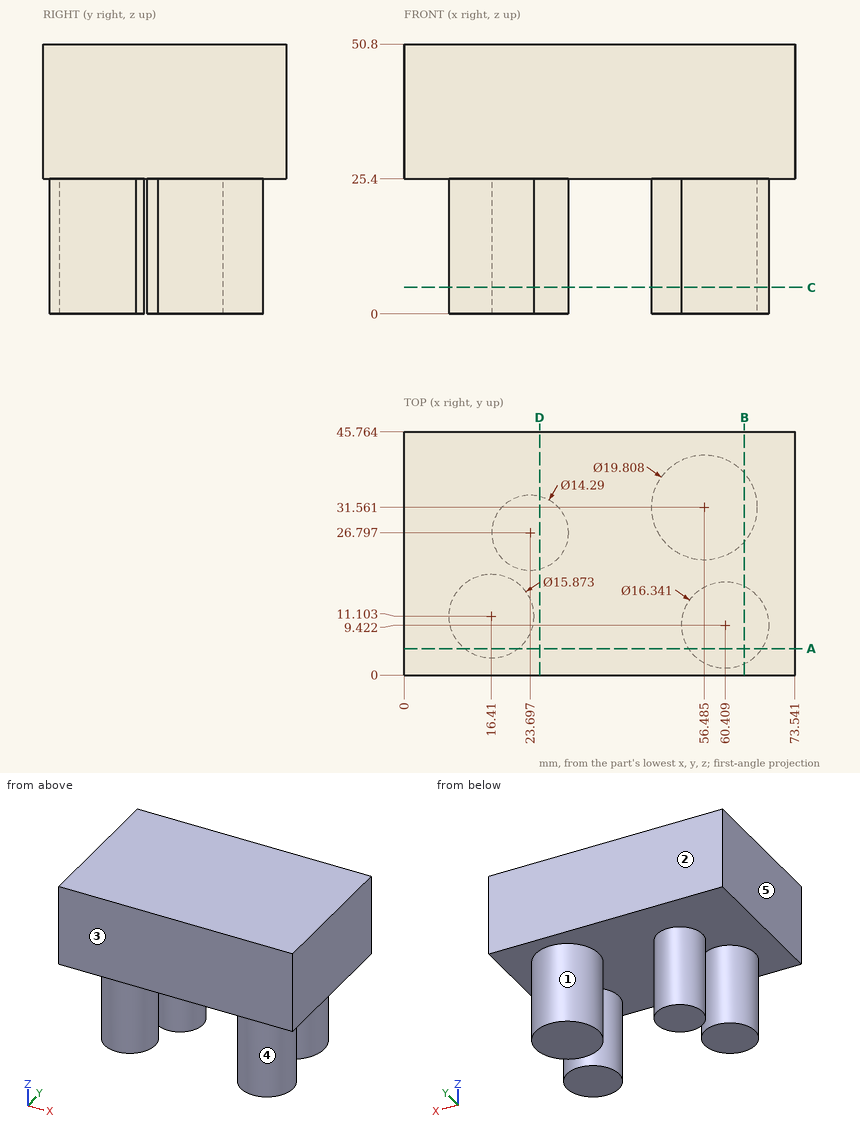
Geometry check sheet. Reference: drawing and pictorial views, mm from the part's lowest x, y, z. A direction names the side the tool comes from. Give positions to 0.01 mm unless a question says otherwise; leave off trailing zeros. Order: outer loops, then holes, each group sorted by start corner. A loop starts at its lowest first (then second) coordinate and runs counter-clockwise, first axis right, second up. Notation, with made-up numbers: M 45.5,-18.5 L 64.5,-18.5 A29 cw 64.5,7.5 Z; hole C 26.5,-10 d4. An arc over 180 degrees is marked long. Answer as a JSON object with one key per item and string values. Group by question number.
1) Scan lines: line 1 along Z through (x, y) = (12.5, 22.5); line 2 along X through (y, z) = (2, 20) (1 decimal); line 3 along X through (y, z) = (32.5, 13.5) (1 decimal). Record each from-to range of solid material in increasing order. Write a range as [from, to].
2) Access from +Z, -Z, +X, -X, +Y, -Y to the whole of each face (thin tool, end or side, straight path). Record for the marked faces 1 and 2.
3) Cross-section at B-B (x = 64). Enter the section's corners in (y, z) (1 decimal), then the cut area to 3 significant figures.
4) Cross-section at A-A (y = 5). Enter the section's corners in (x, z).
5) Depth check by flat-ended pin: pin 1 Ø6 at (y, z) = (11, 8.5) entering from +X; pin 2 Ø10 at (y, z) = (33.5, 10.5) entering from +X; pin 3 Ø12 at (x, z) = (58.5, 15.5) entering from -Y; pin 4 Ø3 at (y, z) = (36, 26.5) entering from -X. Enter the tip coordinate at first touch or a pass-through.
6) Cross-section at C-C (z = 5). Enter the section's corners in (x, y) (1 decimal), then the cut area to 3 significant figures.
7) Cross-section at D-D (x = 25.5). Enter the section's corners in (y, z) (1 decimal), then the cut area to 3 significant figures.
8) Mould release check, pull along X, two halves, no side actions. Record for the marked faces 3, 4 and 5: released by +X, released by -X, zero draft, split by the parting line, or undercut.
Result sheet:
{
 "1": {"line 1": "z = [25.4, 50.8]", "line 2": "x = [57, 63.8]", "line 3": "x = [19.4, 28], [46.6, 66.3]"},
 "2": {"face 1": "-Z", "face 2": "+Z, -Z, +X, -X, +Y"},
 "3": {"outline": "M 0,25.4 L 2.1,25.4 L 2.1,0 L 16.8,0 L 16.8,25.4 L 25.1,25.4 L 25.1,0 L 38,0 L 38,25.4 L 45.8,25.4 L 45.8,50.8 L 0,50.8 Z", "area": "1,860 mm2"},
 "4": {"outline": "M 0,25.4 L 11.34,25.4 L 11.34,0 L 21.48,0 L 21.48,25.4 L 53.54,25.4 L 53.54,0 L 67.28,0 L 67.28,25.4 L 73.54,25.4 L 73.54,50.8 L 0,50.8 Z"},
 "5": {"pin 1": "stops at x = 68.58", "pin 2": "stops at x = 66.39", "pin 3": "stops at y = 1.25", "pin 4": "stops at x = 0"},
 "6": {"outline": "C 16.4,11.1 d15.9; C 23.7,26.8 d14.3; C 56.5,31.6 d19.8; C 60.4,9.4 d16.3", "area": "876 mm2"},
 "7": {"outline": "M 0,25.4 L 19.9,25.4 L 19.9,0 L 33.7,0 L 33.7,25.4 L 45.8,25.4 L 45.8,50.8 L 0,50.8 Z", "area": "1,510 mm2"},
 "8": {"face 3": "zero draft", "face 4": "undercut", "face 5": "released by -X"}
}
